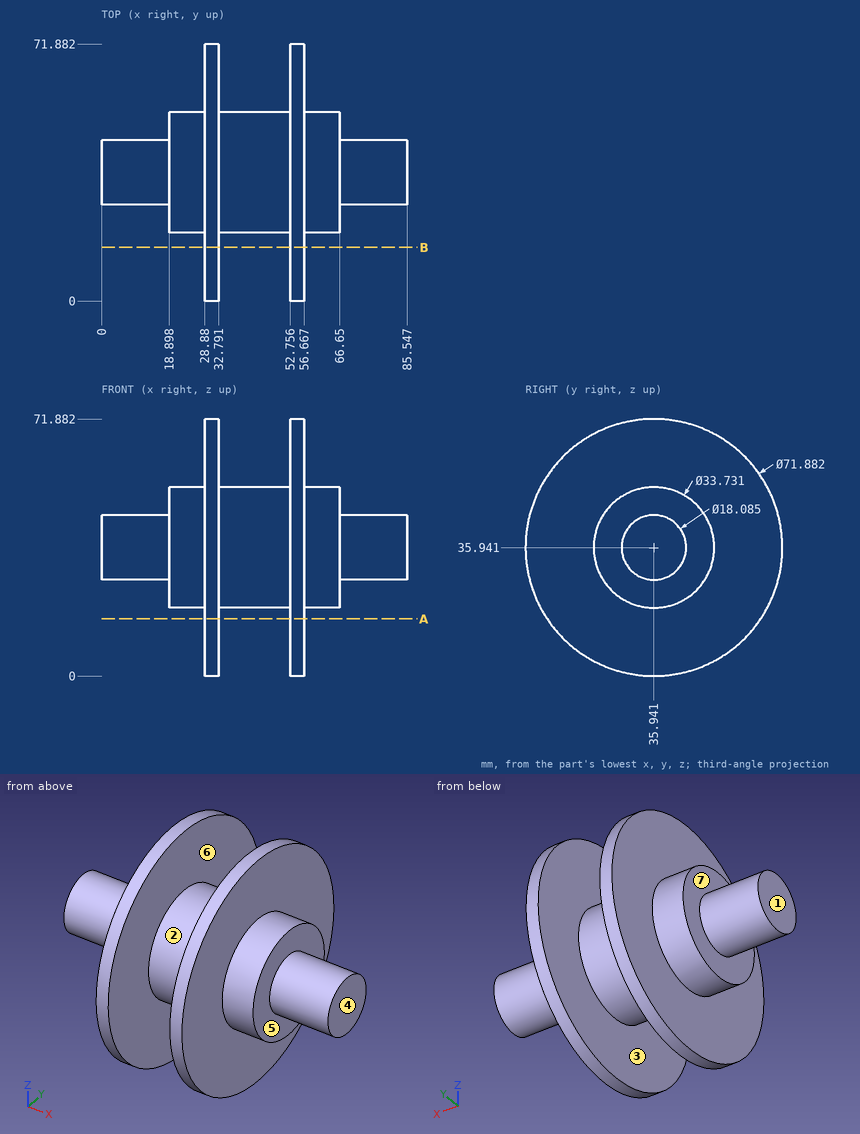
Could you check a few things on this drawing? It's one solid part, dimensions in mm from its lowest x, y, z. A direction names the side the tool comes from. Round coordinates to 2 decimals unless told otherwise and drop trailing zeros. Order: outer loops, then holes, each group sorted by start corner. A loop starts at its lowest first (then second) coordinate and runs counter-clockwise, first axis right, second up.
Q1. Imagine slicing it at B-B, the plane y = 15. List the corners of the cut face in (x, z) for me (1 decimal).
Geometry says:
outline: (28.9, 6.7) - (32.8, 6.7) - (32.8, 65.2) - (28.9, 65.2) - close; (52.8, 6.7) - (56.7, 6.7) - (56.7, 65.2) - (52.8, 65.2) - close
Q2. Imagine slicing it at A-A, the plane z = 16. List the corners of the cut face in (x, y) for me (1 decimal).
Geometry says:
outline: (28.9, 6) - (32.8, 6) - (32.8, 65.8) - (28.9, 65.8) - close; (52.8, 6) - (56.7, 6) - (56.7, 65.8) - (52.8, 65.8) - close
Q3. Which directions (+Z, -Z, +X, -X, +Y, -Y) give clear straight access to the entire face, cutting with the end or side of a thin tool? Please do the marked faces 5, 6 and 7.
Geometry says:
face 5: +X
face 6: none
face 7: -X
Q4. Thinking about a two-plate mould opening in X: for the marked faces 1, 2, 3 and 4, which applies, released by +X, released by -X, zero draft, split by the parting line, or undercut?
Geometry says:
face 1: released by -X
face 2: undercut
face 3: undercut
face 4: released by +X
Q5. Please list where these lines run through material, in increasing order: probe 1 along X at (y, z) = (52, 48) (1 decimal); probe 2 along Y at (x, z) = (29, 37) (1 decimal); probe 3 along X at (y, z) = (49.5, 39).
Geometry says:
probe 1: x = 28.9 to 32.8, 52.8 to 56.7
probe 2: y = 0 to 71.9
probe 3: x = 18.9 to 66.65
Q6. I'm going to push flat-ended pins straight in: P1, Ø2, axis at x = 67, y = 22.5, coming from the -Z side (1 decimal); P2, Ø5, axis at y = 48, z = 39, coming from the +X side; P3, Ø12, axis at x = 38, z = 41, coming from the -Y side. Where does each tip first touch, or does it pass through?
Geometry says:
P1: stops at z = 24.6
P2: stops at x = 66.65
P3: stops at y = 0.06
